The model under review builds one solid part; all positions refer to its coordinate system, in mm. A direction names the side the tool comes from. Round coordinates to 2 decimals unless told otherwise and drop trailing zeros. Order: outer loops, then holes, each group sorted by start corner. A loop starts at its lowest first (then second) coordinate and runs counter-clockwise, first axis right, second up.
Autodesk Fusion 360 part; units mm, degrees
sketch "Sketch1" plane through (0, 0, 0) normal (0, 0, 1) x (1, 0, 0)
  curve L0
  curve L1
  curve L2
  curve L3
sketch "Sketch2" plane through (0, 0, 0) normal (0, 1, 0) x (1, 0, 0)
  circle A0 centre (-0.0361, -7.2532) radius 6.2056
extrude "Extrude2" add sketch "Sketch2" along normal blind 11
hole "Hole1" at (-1.2862, 11, 9.8296) direction (0, -1, 0) diameter 19 depth 3 tip angle 180
hole "Hole2" at (-0.0361, 8, 7.2532) direction (0, -1, 0) diameter 10 depth 7 tip angle 180
sketch "Sketch3" plane through (0, 0, 0) normal (0, 1, 0) x (1, 0, 0)
sketch "Sketch4" plane through (0, 0, 0) normal (0, -1, 0) x (1, 0, 0)
  circle A0 centre (-0.0361, 7.2532) radius 6.2056
  circle A1 centre (-0.0361, 7.2532) radius 4.65
extrude "Extrude4" add sketch "Sketch4" along normal blind 5 contours A1
extrude "Extrude3" [suppressed]
(1) Consider section B-B (x = -4.5). Write out the cut boundary in (y, z).
Data:
outline: (-5, 5.95) - (0, 5.95) - (0, 2.94) - (8, 2.94) - (8, 5) - (1, 5) - (1, 9.51) - (8, 9.51) - (8, 11.56) - (0, 11.56) - (0, 8.56) - (-5, 8.56) - close
(2) For faces 1 (the flat face through (-3, 8, 3)), 2 (the cylindrical face through (-1.54, 4.45, 12.02)), 3 (the cylindrical face through (2.46, -2.46, 3.33)), list the 3-axis set-ups (+Z, -Z, +X, -X, +Y, -Y) from which the entire face can be reached by the end or side of a thin tool; tool diameter is ignored.
Data:
face 1: +Z, -Z, +X, -X, +Y
face 2: +Y
face 3: -Y
(3) Consider section C-C (y = 4.75). Write out the cut boundary in (x, z).
Data:
outline: circle Ø12.41 at (-0.04, 7.25); hole circle Ø10 at (-0.04, 7.25)
(4) Draft analysis for pull direction X (two halves, no side actions). For faces 4 (the cylindrical face through (-1.4, 3.9, 1.2)), 5 (the flat face through (0, -5, 7)), 6 (the flat face through (0, 1, 7)), state which applies: pulls with the +X half, pulls with the -X half, needs draft (parallel to the pull), parting line crosses it, or undercut.
Data:
face 4: parting line crosses it
face 5: needs draft
face 6: undercut
(5) Consider section A-A (z = 8). Write out the cut boundary in (x, y), and give its area (3 significant figures).
Data:
outline: (-6.2, 0) - (-4.63, 0) - (-4.63, -5) - (4.55, -5) - (4.55, 0) - (6.12, 0) - (6.12, 8) - (4.91, 8) - (4.91, 1) - (-4.98, 1) - (-4.98, 8) - (-6.2, 8) - close
area: 75.2 mm2
(6) Consider section D-D (x = 5.5). Write out the cut boundary in (y, z), and give its area (3 significant figures).
Data:
outline: (0, 4.45) - (8, 4.45) - (8, 10.06) - (0, 10.06) - close
area: 44.9 mm2
(7) Insertion check: pin 1 (3 mm diameter, centred on x = 2, z = 8.5, fed in from +Y); pin 2 (4 mm diameter, centred on x = -3, y = -3.5, fed in from -Z); pin 3 (3 mm diameter, centred on x = -1.5, y = 1.5, fed in from +Z); pin 4 (2 mm diameter, centred on y = 2, z = 3, fed in from +X). Each pin has a flat end and moves straight along its axis. Give the tip position at first contact, or say it passes through.
Data:
pin 1: stops at y = 1
pin 2: stops at z = 2.7
pin 3: stops at z = 13.46
pin 4: stops at x = 5.25
(8) To check wall thickness, follow probe 1 along Z at (x, y) = (0, 7); probe 2 along Y at (x, z) = (1.5, 6); probe 3 along Y at (x, z) = (-2.25, 2.5). State the ranges of each line that lie inside material, in increasing order.
Data:
probe 1: z = 1.05 to 2.25, 12.25 to 13.46
probe 2: y = -5 to 1
probe 3: y = 0 to 8
